from build123d import *

# Parameters (mm, degrees)
F0_R     = 2.75
F1_DEPTH = 25
F2_SIZE  = 1
F4_DEPTH = 5
F5_R     = 0.5


with BuildPart() as f1:
    # F0 (on Front) → F1 (new body)
    with BuildSketch(Plane.XZ):
        Circle(F0_R)
    extrude(amount=-F1_DEPTH)

    # F2
    f2_edges = [f1.edges().sort_by_distance(p)[0] for p in [
        (-2.75, 25, 0),
    ]]
    chamfer(f2_edges, length=F2_SIZE)

    # F3 (on face) → F4 (join)
    with BuildSketch(Plane.XZ):
        Polygon((5, -2.886751), (5, 2.886751), (0, 5.773503), (-5, 2.886751), (-5, -2.886751), (0, -5.773503), align=None)
    extrude(amount=F4_DEPTH)

    # F5
    f5_edges = [f1.edges().sort_by_distance(p)[0] for p in [
        (5, -2.5, 2.886751),
        (0, -2.5, 5.773503),
        (-5, -2.5, 2.886751),
        (0, -2.5, -5.773503),
        (-5, -2.5, -2.886751),
        (5, -2.5, -2.886751),
    ]]
    fillet(f5_edges, radius=F5_R)

    # F6 (on Right) → F7 (revolve, cut)
    with BuildSketch(Plane.YZ):
        Polygon((-5.362704, 6), (-5.362704, 3.8), (-4, 6), align=None)
    revolve(axis=Axis((0, -4.871394, 0), (0, 1, 0)), mode=Mode.SUBTRACT)


solid = f1.part
Geometry: final body of the model. Coordinates: model frame, mm. A direction names the side the tool comes from. Give positions to 0.01 mm unless a question says otherwise; leave off trailing zeros. Write each loop counter-clockwise with the first axis right and the second up, starting at its lowest first coordinate (ties: lowest second). Pieces come first, ordered by that corner, then holes.
(1) Cut plane A-A, the plane z = 0. Return loops of the section in (x, y), then the cut area to 3 significant figures.
(2) First-contact query: P1, Ø1, axis at y = 16.5, z = -1, coming from the +X side; P2, Ø6, axis at x = 0, y = 18, coming from the +Z side. Flat tips, straight axial feed; report the tip coordinate or a pass-through.
(3) Ray query, line 1 (Y direction, x = 2.75, z = 0.5); line 2 (X direction, y = 20, z = 0.5); line 3 (X direction, y = 21, z = -1.25). Return the intervals inside material, ascending.
(4) Cut plane B-B, the plane y = 1. Return loops of the section in (x, z).
(5) Access query for faces 1 (the flat face through (0, 25, 0)), 2 (the cylindrical face through (-0.596, 11.832, -2.685)). Directions: +Z, -Z, +X, -X, +Y, -Y. A direction counts if a zero-diameter tool reaches every point of the face in a straight line with its end or side. Return the directions, or none.
Values follow:
1. outline: (-5, -4.62) - (-4.39, -5) - (4.39, -5) - (5, -4.62) - (5, 0) - (2.75, 0) - (2.75, 24) - (1.75, 25) - (-1.75, 25) - (-2.75, 24) - (-2.75, 0) - (-5, 0) - close
1. area: 186 mm2
2. P1: stops at x = 2.7
2. P2: stops at z = 2.75
3. line 1: y = -5 to 0
3. line 2: x = -2.7 to 2.7
3. line 3: x = -2.45 to 2.45
4. outline: circle Ø5.5 at (0, 0)
5. face 1: +Z, -Z, +X, -X, +Y
5. face 2: +Y
